Autodesk Inventor part; units mm, degrees
ref_plane "to_body_XY" through (6.5, 15.3, 228.6) normal (0, 0, 1) x (1, 0, 0)
ref_plane "to_body_YZ" through (6.5, 15.3, 228.6) normal (1, 0, 0) x (0, 1, 0)
ref_plane "to_body_ZX" through (6.5, 15.3, 228.6) normal (0, 1, 0) x (0, 0, 1)
sketch "Sketch_1" plane through (0, 0, 0) normal (0, 0, 1) x (1, 0, 0)
  arc A0 (1.8281, 29.2788) -> (4.2342, 27.8447) centre (3.65, 29.6) ccw
  arc A1 (5.55, 26.8958) -> (4.2342, 27.8447) centre (4.55, 26.8958) ccw
  line L0 (5.55, 26.8958) -> (5.55, 3.7042)
  arc A2 (4.2342, 2.7553) -> (5.55, 3.7042) centre (4.55, 3.7042) ccw
  arc A3 (4.2342, 2.7553) -> (1.8281, 1.3212) centre (3.65, 1) ccw
  line L1 (1.8281, 1.3212) -> (2.2787, 1.2418)
  arc A4 (4.8691, 1.3916) -> (2.2787, 1.2418) centre (3.65, 0) ccw
  arc A5 (4.8691, 1.3916) -> (6.3379, 1.5571) centre (5.528, 2.1437) ccw
  line L2 (6.3379, 1.5571) -> (6.55, 1.85)
  line L3 (6.55, 1.85) -> (6.55, 28.75)
  line L4 (6.55, 28.75) -> (6.3379, 29.0429)
  arc A6 (6.3379, 29.0429) -> (4.8691, 29.2084) centre (5.528, 28.4563) ccw
  arc A7 (2.2787, 29.3582) -> (4.8691, 29.2084) centre (3.65, 30.6) ccw
  line L5 (2.2787, 29.3582) -> (1.8281, 29.2788)
extrude "Extrusion1" add sketch "Sketch_1" along normal blind 457.2
sketch "Sketch2" plane through (6.55, 1.85, 0) normal (1, 0, 0) x (0, 0, -1)
  point P0 (-415.2, 13.45)
hole "Hole1" at (6.55, 15.3, 415.2) direction (-1, 0, 0) diameter 9.5 depth 1
sketch "Sketch_5" plane through (6.55, 0, 0) normal (1, 0, 0) x (0, 0, -1)
  line L0 (-434.05, 15.7) -> (-434.05, 14.9)
  arc A0 (-434.05, 14.9) -> (-431.8, 12.65) centre (-431.8, 14.9) ccw
  arc A1 (-431.8, 12.65) -> (-429.55, 14.9) centre (-431.8, 14.9) ccw
  line L1 (-429.55, 14.9) -> (-429.55, 15.7)
  arc A2 (-429.55, 15.7) -> (-431.8, 17.95) centre (-431.8, 15.7) ccw
  arc A3 (-431.8, 17.95) -> (-434.05, 15.7) centre (-431.8, 15.7) ccw
extrude "Extrusion2" cut sketch "Sketch_5" against normal blind 1
sketch "Sketch_6" plane through (6.55, 0, 0) normal (1, 0, 0) x (0, 0, -1)
  line L0 (-27.65, 15.7) -> (-27.65, 14.9)
  arc A0 (-27.65, 14.9) -> (-25.4, 12.65) centre (-25.4, 14.9) ccw
  arc A1 (-25.4, 12.65) -> (-23.15, 14.9) centre (-25.4, 14.9) ccw
  line L1 (-23.15, 14.9) -> (-23.15, 15.7)
  arc A2 (-23.15, 15.7) -> (-25.4, 17.95) centre (-25.4, 15.7) ccw
  arc A3 (-25.4, 17.95) -> (-27.65, 15.7) centre (-25.4, 15.7) ccw
extrude "Extrusion3" cut sketch "Sketch_6" against normal blind 1
sketch "Sketch_7" plane through (6.55, 0, 0) normal (1, 0, 0) x (0, 0, -1)
  arc A0 (-332.85, 15.3) -> (-330.6, 13.05) centre (-330.6, 15.3) ccw
  line L0 (-330.6, 13.05) -> (-329.8, 13.05)
  arc A1 (-329.8, 13.05) -> (-327.55, 15.3) centre (-329.8, 15.3) ccw
  arc A2 (-327.55, 15.3) -> (-329.8, 17.55) centre (-329.8, 15.3) ccw
  line L1 (-329.8, 17.55) -> (-330.6, 17.55)
  arc A3 (-330.6, 17.55) -> (-332.85, 15.3) centre (-330.6, 15.3) ccw
extrude "Extrusion4" cut sketch "Sketch_7" against normal blind 1
sketch "Sketch_8" plane through (6.55, 0, 0) normal (1, 0, 0) x (0, 0, -1)
  arc A0 (-231.25, 15.3) -> (-229, 13.05) centre (-229, 15.3) ccw
  line L0 (-229, 13.05) -> (-228.2, 13.05)
  arc A1 (-228.2, 13.05) -> (-225.95, 15.3) centre (-228.2, 15.3) ccw
  arc A2 (-225.95, 15.3) -> (-228.2, 17.55) centre (-228.2, 15.3) ccw
  line L1 (-228.2, 17.55) -> (-229, 17.55)
  arc A3 (-229, 17.55) -> (-231.25, 15.3) centre (-229, 15.3) ccw
extrude "Extrusion5" cut sketch "Sketch_8" against normal blind 1
sketch "Sketch_9" plane through (6.55, 0, 0) normal (1, 0, 0) x (0, 0, -1)
  arc A0 (-129.65, 15.3) -> (-127.4, 13.05) centre (-127.4, 15.3) ccw
  line L0 (-127.4, 13.05) -> (-126.6, 13.05)
  arc A1 (-126.6, 13.05) -> (-124.35, 15.3) centre (-126.6, 15.3) ccw
  arc A2 (-124.35, 15.3) -> (-126.6, 17.55) centre (-126.6, 15.3) ccw
  line L1 (-126.6, 17.55) -> (-127.4, 17.55)
  arc A3 (-127.4, 17.55) -> (-129.65, 15.3) centre (-127.4, 15.3) ccw
extrude "Extrusion6" cut sketch "Sketch_9" against normal blind 1
ref_plane "to_body_XY" through (6.5, 15.3, 228.6) normal (0, 0, 1) x (1, 0, 0)
ref_plane "to_body_YZ" through (6.5, 15.3, 228.6) normal (1, 0, 0) x (0, 1, 0)
ref_plane "to_body_ZX" through (6.5, 15.3, 228.6) normal (0, 1, 0) x (0, 0, 1)
ref_plane "to_slider_XY" through (6.5, 15.3, 228.6) normal (0, 0, 1) x (1, 0, 0)
ref_plane "to_slider_YZ" through (6.5, 15.3, 228.6) normal (1, 0, 0) x (0, 1, 0)
ref_plane "to_slider_ZX" through (6.5, 15.3, 228.6) normal (0, 1, 0) x (0, 0, 1)
properties part number "rail_SSRN3618" material "鉄 灰色"
Here's how the part is built. I have some questions about the finished solid (model axes, mm). Round coordinates to 2 decimals unless told otherwise and drop trailing zeros. Write each loop counter-clockwise with the first axis right and the second up, starting at its lowest first coordinate (ties: lowest second). Pieces come first, ordered by that corner, then holes.
1. Suppose I cut it at A-A (z = 288). List the corners of the cut face in (x, y) for me, and give its area (3 significant figures).
2. If we mould it in two halves opening along Y, with no side actions, what happens to faces 1 (the flat face through (5.55, 15, 225)), 2 (the flat face through (6.55, 15, 225))? For each: released by +Y, released by -Y, zero draft, split by the parting line, or undercut.
3. Suppose I cut it at B-B (z = 415.2). List the corners of the cut face in (x, y) for me.
4. Will these pins go through, and if not, where does the flat tip stop? pin 1 Ø7 at (y, z) = (19, 225) entering from -X; pin 2 Ø0.6 at (x, z) = (6, 229) entering from -Y.
5. I need wall thicknesses on L1, parallel to Y at x = 6.1, z = 415.2; L2, parallel to Y at x = 6.35, z = 415.2; L3, parallel to Y at x = 6.15, z = 218. Which ranges of each line are inside material? Lowest first, please.
Answer sheet:
1. outline: (1.83, 1.32) - (2.28, 1.24) arc R1.85 cw to (4.87, 1.39) arc R1 ccw to (6.34, 1.56) - (6.55, 1.85) - (6.55, 28.75) - (6.34, 29.04) arc R1 ccw to (4.87, 29.21) arc R1.85 cw to (2.28, 29.36) - (1.83, 29.28) arc R1.85 ccw to (4.23, 27.84) arc R1 cw to (5.55, 26.9) - (5.55, 3.7) arc R1 cw to (4.23, 2.76) arc R1.85 ccw to start
1. area: 36.2 mm2
2. face 1: undercut
2. face 2: zero draft
3. outline: (1.83, 1.32) - (2.28, 1.24) arc R1.85 cw to (4.87, 1.39) arc R1 ccw to (6.34, 1.56) - (6.55, 1.85) - (6.55, 10.55) - (5.55, 10.55) - (5.55, 3.7) arc R1 cw to (4.23, 2.76) arc R1.85 ccw to start; (1.83, 29.28) arc R1.85 ccw to (4.23, 27.84) arc R1 cw to (5.55, 26.9) - (5.55, 20.05) - (6.55, 20.05) - (6.55, 28.75) - (6.34, 29.04) arc R1 ccw to (4.87, 29.21) arc R1.85 cw to (2.28, 29.36) - close
4. pin 1: stops at x = 5.55
4. pin 2: stops at y = 1.16
5. L1: y = 1.32 to 10.55, 20.05 to 29.28
5. L2: y = 1.57 to 10.55, 20.05 to 29.03
5. L3: y = 1.36 to 29.24
